Read the model definition and answer for the solid it produces. Units are mm, in the model's axes. A direction names the side the tool comes from. Round coordinates to 2 decimals unless told otherwise and drop trailing zeros. One line per item, written item: value. Start each with the question number.
1. Section A-A (x = -25) is taken. State how many separate pieces and enclosed holes the cut face has, then the cut area to 3 significant figures.
2. Flat-ended cylindrical pins translate along their axes: pin 1 Ø2.5 at (x, z) = (-34.46, -19.25) entering from -Y; pin 2 Ø1.7 at (x, z) = (1.5, -3) entering from +Y; pin 3 Ø2 at (y, z) = (-4.5, 1) entering from +X; pin 4 Ø1 at (x, z) = (-2.5, 2.5) entering from +Y. Find the tip coordinate at first contact, or state that the pin passes through.
3. The mould has two halves that part along X. Classify faces 1 (the face through (-14.74, 1.48, -10.33)), 2 (the face through (2.64, -5.27, -59.94)): released by +X, released by -X, zero draft, split by the parting line, or undercut.
4. Consider line 1 (Z direction, x = 30, y = -2.5); line 2 (Z direction, x = -33, y = -5); line 3 (Y direction, x = 11, z = -12). Determine where each line is inside the solid, lowest interval first.
5. For faces 3 (the face through (16.42, 1.48, -19.57)), 4 (the face through (3.3, 0.7, 2.9)), determine the directions among +Z, -Z, +X, -X, +Y, -Y from which every point of the face is accessible in a straight line to the end or side of a thin tool.
from build123d import *

# Parameters (mm, degrees)
SKETCH1_R           = 60
SKETCH1_R_2         = 4.15
SKETCH1_R_3         = 0.6
BOSS_EXTRUDE1_DEPTH = 3
BOSS_EXTRUDE2_START = -6.5
SKETCH1_5_R         = 60
SKETCH1_5_R_2       = 56.4
SKETCH1_5_R_3       = 40.6
SKETCH1_5_R_4       = 37
BOSS_EXTRUDE2_DEPTH = 6.5
FILLET1_R           = 8
CHAMFER1_SIZE       = 7
CUT_EXTRUDE1_START  = -2.1
CUT_EXTRUDE1_DEPTH  = 2.1
SKETCH3_R           = 2
CUT_EXTRUDE2_DEPTH  = 5
FILLET2_R           = 5
CUT_EXTRUDE4_START  = -0.2
CUT_EXTRUDE4_DEPTH  = 0.2


with BuildPart() as part:
    # Sketch1 → Boss-Extrude1 (new body)
    with BuildSketch(Plane(origin=(0, 0, 0), x_dir=(1, 0, 0), z_dir=(0, 1, 0))):
        with Locations(Location((0, 0, 0), (0, 0, 270))):
            Circle(SKETCH1_R)
        with Locations(Location((0, 0, 0), (0, 0, 270))):
            Circle(SKETCH1_R_2, mode=Mode.SUBTRACT)
        with Locations(Location((-11, 0, 0), (0, 0, 270))):
            Circle(SKETCH1_R_3, mode=Mode.SUBTRACT)
        with Locations(Location((11, 0, 0), (0, 0, 270))):
            Circle(SKETCH1_R_3, mode=Mode.SUBTRACT)
        with BuildLine():
            Line((-11.570176974, 13.788799976), (-21.143111218, 25.197378752))
            ThreePointArc((-21.143111218, 25.197378752), (-26.867310164, 18.975950371), (-30.816661277, 11.500975423))
            Line((-30.816661277, 11.500975423), (-16.863848516, 6.293696309))
            ThreePointArc((-16.863848516, 6.293696309), (-14.702639088, 10.384238241), (-11.570176974, 13.788799976))
        make_face(mode=Mode.SUBTRACT)
        with BuildLine():
            Line((-8.872947439, 15.661123962), (-16.214247626, 28.618826354))
            ThreePointArc((-16.214247626, 28.618826354), (-8.384047872, 31.806395414), (0, 32.892841895))
            Line((0, 32.892841895), (0, 18))
            ThreePointArc((0, 18), (-4.588015295, 17.405462236), (-8.872947439, 15.661123962))
        make_face(mode=Mode.SUBTRACT)
        with BuildLine():
            Line((3.269704356, 17.700537659), (5.974992691, 32.345610371))
            ThreePointArc((5.974992691, 32.345610371), (14.022203597, 29.754274554), (21.143111218, 25.197378752))
            Line((21.143111218, 25.197378752), (11.570176974, 13.788799976))
            ThreePointArc((11.570176974, 13.788799976), (7.673391845, 16.28247701), (3.269704356, 17.700537659))
        make_face(mode=Mode.SUBTRACT)
        with BuildLine():
            Line((13.882425145, 11.457673066), (25.368467523, 20.937523814))
            ThreePointArc((25.368467523, 20.937523814), (29.867310164, 13.779797948), (32.393125717, 5.711782053))
            Line((32.393125717, 5.711782053), (17.726539554, 3.125667198))
            ThreePointArc((17.726539554, 3.125667198), (16.34433366, 7.540739832), (13.882425145, 11.457673066))
        make_face(mode=Mode.SUBTRACT)
        with BuildLine():
            Line((15.588457268, -9), (28.486036684, -16.446420948))
            ThreePointArc((28.486036684, -16.446420948), (31.737170367, -8.642399263), (32.891754462, -0.26746283))
            Line((32.891754462, -0.26746283), (17.999404922, -0.146364092))
            ThreePointArc((17.999404922, -0.146364092), (17.367580109, -4.72939332), (15.588457268, -9))
        make_face(mode=Mode.SUBTRACT)
        with BuildLine():
            Line((13.694263095, -11.681915865), (25.024623937, -21.347300644))
            ThreePointArc((25.024623937, -21.347300644), (18.756855836, -27.020721809), (11.250014499, -30.909160806))
            Line((11.250014499, -30.909160806), (6.15636258, -16.914467174))
            ThreePointArc((6.15636258, -16.914467174), (10.264342805, -14.786590776), (13.694263095, -11.681915865))
        make_face(mode=Mode.SUBTRACT)
        with BuildLine():
            Line((2.981423371, -17.751369375), (5.448193754, -32.438499237))
            ThreePointArc((5.448193754, -32.438499237), (-3, -32.755748319), (-11.250014499, -30.909160806))
            Line((-11.250014499, -30.909160806), (-6.15636258, -16.914467174))
            ThreePointArc((-6.15636258, -16.914467174), (-1.641694572, -17.924978073), (2.981423371, -17.751369375))
        make_face(mode=Mode.SUBTRACT)
        with BuildLine():
            Line((-9.126457483, -15.51475987), (-16.677506836, -28.351363524))
            ThreePointArc((-16.677506836, -28.351363524), (-23.353122495, -23.163996151), (-28.486036684, -16.446420948))
            Line((-28.486036684, -16.446420948), (-15.588457268, -9))
            ThreePointArc((-15.588457268, -9), (-12.779564814, -12.676068916), (-9.126457483, -15.51475987))
        make_face(mode=Mode.SUBTRACT)
        with BuildLine():
            Line((-16.963967452, -6.018621794), (-30.999616628, -10.998309728))
            ThreePointArc((-30.999616628, -10.998309728), (-32.779059433, -2.733552745), (-32.393125717, 5.711782053))
            Line((-32.393125717, 5.711782053), (-17.726539554, 3.125667198))
            ThreePointArc((-17.726539554, 3.125667198), (-17.93773465, -1.495886234), (-16.963967452, -6.018621794))
        make_face(mode=Mode.SUBTRACT)
    extrude(amount=BOSS_EXTRUDE1_DEPTH)

    # Sketch1<5> → Boss-Extrude2 (add)
    # profile 1 of 2: a face of its own
    with BuildSketch(Plane(origin=(0, 0, 0), x_dir=(1, 0, 0), z_dir=(0, 1, 0)).offset(BOSS_EXTRUDE2_START)):
        with Locations(Location((0, 0, 0), (0, 0, 270))):
            Circle(SKETCH1_5_R)
        with Locations(Location((0, 0, 0), (0, 0, 270))):
            Circle(SKETCH1_5_R_2, mode=Mode.SUBTRACT)
    # profile 2 of 2: a face of its own
    with BuildSketch(Plane(origin=(0, 0, 0), x_dir=(1, 0, 0), z_dir=(0, 1, 0)).offset(BOSS_EXTRUDE2_START)):
        with Locations(Location((0, 0, 0), (0, 0, 270))):
            Circle(SKETCH1_5_R_3)
        with Locations(Location((0, 0, 0), (0, 0, 270))):
            Circle(SKETCH1_5_R_4, mode=Mode.SUBTRACT)
    extrude(amount=BOSS_EXTRUDE2_DEPTH)

    # Fillet1
    # the kernel refuses this fillet: 8 mm, written as the material it adds along each edge
    with BuildSketch(Plane(origin=(0, 0, 0), x_dir=(0, 0, 1), z_dir=(-1, 0, 0))) as fillet1_piece_1:
        with BuildLine():
            CenterArc((48.541883177, -8), FILLET1_R, 10.806922875, 79.193077125)
            Line((48.541883177, 0), (48.541883177, 0.16))
            Line((48.541883177, 0.16), (56.4, 0.16))
            Line((56.4, 0.16), (56.56, 0))
            ThreePointArc((56.56, 0), (56.56, -3.25), (56.557162336, -6.47))
            Line((56.557162336, -6.47), (56.4, -6.5))
        make_face()
    revolve(axis=Axis((0, 0, 0), (0, 1, 0)))
    with BuildSketch(Plane(origin=(0, 0, 0), x_dir=(0, 0, 1), z_dir=(-1, 0, 0))) as fillet1_piece_2:
        with BuildLine():
            CenterArc((48.458116823, -8), FILLET1_R, 90, 79.193077125)
            Line((40.6, -6.5), (40.442837664, -6.47))
            ThreePointArc((40.442837664, -6.47), (40.44, -3.25), (40.44, 0))
            Line((40.44, 0), (40.6, 0.16))
            Line((40.6, 0.16), (48.458116823, 0.16))
            Line((48.458116823, 0.16), (48.458116823, 0))
        make_face()
    revolve(axis=Axis((0, 0, 0), (0, 1, 0)))

    # Chamfer1
    chamfer1_edges = [part.edges().sort_by_distance(p)[0] for p in [
        (0, 3, -60),
    ]]
    chamfer(chamfer1_edges, length=CHAMFER1_SIZE)

    # Sketch2 → Cut-Extrude1 (cut)
    with BuildSketch(Plane(origin=(0, 3, 0), x_dir=(1, 0, 0), z_dir=(0, 1, 0)).offset(CUT_EXTRUDE1_START)):
        with BuildLine():
            Line((0.712064808, -4.088454929), (15, -1.6))
            ThreePointArc((15, -1.6), (16.6, 0), (15, 1.6))
            Line((15, 1.6), (0.712064808, 4.088454929))
            ThreePointArc((0.712064808, 4.088454929), (0, 4.15), (-0.712064808, 4.088454929))
            Line((-0.712064808, 4.088454929), (-15, 1.6))
            ThreePointArc((-15, 1.6), (-16.6, 0), (-15, -1.6))
            Line((-15, -1.6), (-0.712064808, -4.088454929))
            ThreePointArc((-0.712064808, -4.088454929), (0, -4.15), (0.712064808, -4.088454929))
        make_face()
    extrude(amount=CUT_EXTRUDE1_DEPTH, mode=Mode.SUBTRACT)

    # Sketch3 → Cut-Extrude2 (cut)
    with BuildSketch(Plane(origin=(0, 3, 0), x_dir=(1, 0, 0), z_dir=(0, 1, 0))):
        with Locations(Location((-34.458294856, -19.25, 0), (0, 0, 270))):
            Circle(SKETCH3_R)
        with Locations(Location((-34.458294856, 19.25, 0), (0, 0, 270))):
            Circle(SKETCH3_R)
        with Locations(Location((34.458294856, 19.25, 0), (0, 0, 270))):
            Circle(SKETCH3_R)
        with Locations(Location((34.458294856, -19.25, 0), (0, 0, 270))):
            Circle(SKETCH3_R)
    extrude(amount=-CUT_EXTRUDE2_DEPTH, mode=Mode.SUBTRACT)

    # Fillet2
    fillet2_edges = [part.edges().sort_by_distance(p)[0] for p in [
        (0, -6.5, -56.4),
        (0, -6.5, -40.6),
    ]]
    fillet(fillet2_edges, radius=FILLET2_R)

    # Sketch4 → Cut-Extrude4 (cut)
    with BuildSketch(Plane(origin=(0, 0.9, 0), x_dir=(1, 0, 0), z_dir=(0, 1, 0)).offset(CUT_EXTRUDE4_START)):
        with BuildLine():
            ThreePointArc((-4.15, -1e-08), (-3.1762847, 2.670901627), (-0.712064808, 4.088454929))
            Line((-0.712064808, 4.088454929), (-4.15, 3.489687741))
            Line((-4.15, 3.489687741), (-4.15, -1e-08))
        make_face()
        with BuildLine():
            ThreePointArc((-0.712064808, -4.088454929), (-3.176284694, -2.670901635), (-4.15, -1e-08))
            Line((-4.15, -1e-08), (-4.15, -3.489687741))
            Line((-4.15, -3.489687741), (-0.712064808, -4.088454929))
        make_face()
        with BuildLine():
            ThreePointArc((0.712064808, 4.088454929), (3.176284696, 2.670901632), (4.15, 3e-09))
            Line((4.15, 3e-09), (4.15, 3.489687741))
            Line((4.15, 3.489687741), (0.712064808, 4.088454929))
        make_face()
        with BuildLine():
            ThreePointArc((4.15, 3e-09), (3.176284698, -2.67090163), (0.712064808, -4.088454929))
            Line((0.712064808, -4.088454929), (4.15, -3.489687741))
            Line((4.15, -3.489687741), (4.15, 3e-09))
        make_face()
    extrude(amount=CUT_EXTRUDE4_DEPTH, mode=Mode.SUBTRACT)


solid = part.part
Answer:
1. separate pieces: 4
1. enclosed holes: 0
1. area: 341 mm^2
2. pin 1: y = -6.39
2. pin 2: y = 0.7
2. pin 3: x = 60
2. pin 4: through
3. face 1: undercut
3. face 2: split by the parting line
4. line 1: -50.22 to -45.32, -30.31 to -21.66, 21.66 to 30.31, 45.32 to 50.22
4. line 2: -50.11 to -45.53, -23.94 to -16.73, 16.73 to 23.94, 45.53 to 50.11
4. line 3: 0 to 3
5. face 3: +Y, -Y
5. face 4: +Y
